Design review of the part built by this model. Coordinates are the model's own, in mm. A direction names the side the tool comes from. Coordinates: 2 decimals unless noted, no trailing zeros. Loops run counter-clockwise (first coordinate to the right, second up) from the corner with the lowest first, then second, coordinate; pieces in that order, holes last. Notation, with made-up numbers: (14, -7.75) -> (72, -7.75) arc R18 ccw to (72, -1.75) -> close; hole circle Ø4 at (1, 83). An arc over 180 degrees is marked (long way). Use CSV: the item, a comma, the result in double quotes.
```python
from build123d import *

# Parameters (mm, degrees)
SKETCH1_R           = 1.5
BOSS_EXTRUDE1_DEPTH = 13
SKETCH2_R           = 2.5
BOSS_EXTRUDE2_DEPTH = 2
FILLET1_R           = 1.5
CUT_EXTRUDE1_DEPTH  = 1.2


with BuildPart() as part:
    # Sketch1 → Boss-Extrude1 (new body)
    with BuildSketch(Plane.XY):
        with Locations(Location((0, 0, 0), (0, 0, 180))):
            Circle(SKETCH1_R)
    extrude(amount=BOSS_EXTRUDE1_DEPTH)

    # Sketch2 → Boss-Extrude2 (add)
    with BuildSketch(Plane.XY.offset(13)):
        Circle(SKETCH2_R)
    extrude(amount=BOSS_EXTRUDE2_DEPTH)

    # Fillet1
    fillet1_edges = [part.edges().sort_by_distance(p)[0] for p in [
        (-2.5, 0, 15),
    ]]
    fillet(fillet1_edges, radius=FILLET1_R)

    # Sketch3 → Cut-Extrude1 (cut)
    with BuildSketch(Plane.XY.offset(15)):
        Polygon((2.5, 0), (0.58177786, 0.58177786), (0, 2.5), (-0.58177786, 0.58177786), (-2.5, 0), (-0.58177786, -0.58177786), (0, -2.5), (0.58177786, -0.58177786), align=None)
    extrude(amount=-CUT_EXTRUDE1_DEPTH, mode=Mode.SUBTRACT)


solid = part.part
```
Item 1: To check wall thickness, follow line 1 along Z through (x, y) = (1.3, -0.05); line 2 along X through (y, z) = (0.1, 11.5). State the ranges of each line that lie inside material, in increasing order.
Checked values:
line 1,"0 to 13.8"
line 2,"-1.5 to 1.5"
Item 2: Machinability: for faces 1 (the face through (-0.363, -1.303, 14.275)), 2 (the face through (0, -2, 13)), which of the approach directions +Z, -Z, +X, -X, +Y, -Y give a long, thin tool a straight path to every point of the face, cutting with its end or side? Answer none if there is none.
Checked values:
face 1,"+Z"
face 2,"-Z"
Item 3: Add section A-A (z = 2). Give the boundary of the cut face in (x, y).
Checked values:
outline,"circle Ø3 at (0, 0)"
Item 4: Clearance check with flat-ended pins moving along their axes: pin 1 (1 mm diameter, centred on y = 1, z = 11.5, fed in from -X); pin 2 (1.5 mm diameter, centred on y = -1, z = 8.5, fed in from +X). State where each tip first meets the part, or that it passes through.
Checked values:
pin 1,"x = -1.41"
pin 2,"x = 1.48"
Item 5: Draft analysis for pull direction X (two halves, no side actions). For faces 3 (the face through (-0.54, -2.44, 13.25)), 4 (the face through (0.355, -1.329, 14.275)), 5 (the face through (0, 0, 0)), state which applies: pulls with the +X half, pulls with the -X half, needs draft (parallel to the pull), parting line crosses it, or undercut.
Checked values:
face 3,"parting line crosses it"
face 4,"undercut"
face 5,"needs draft"
